The listing builds one solid part. Answer for the finished solid, in the listing's coordinates (mm). Coordinates: 2 decimals unless noted, no trailing zeros. Order: outer loops, then holes, each group sorted by start corner. A loop starts at its lowest first (then second) coordinate and runs counter-clockwise, first axis right, second up. Notation, with made-up numbers: (18, -10) - (35, -10) arc R27 ccw to (35, 16) - close; hole circle Ø11 at (-35.5, -16.5). An arc over 180 degrees is marked (long way). Use a Markdown table: item, result. Add a question column.
Item 1: The part is cut by section A-A, the plane z = -15.5. Give the vertices of the cut face in (x, y) (3 decimals), then the cut area to 3 significant figures.
Item 2: Find the intervals of material crossed by line 1 along Y through (x, z) = (-18, -4); line 2 along X through (y, z) = (-2.5, 0.5) (3 decimals); line 3 along X through (y, z) = (-10.5, 14.5) (3 decimals), in increasing order.
Item 3: The part is cut by section B-B, the plane x = -15. Give the vertices of the cut face in (y, z) (3 decimals), then the cut area to 3 significant figures.
Item 4: Flat-ended cylindrical pins translate along their axes: P1, Ø1.5, axis at x = -9.5, z = -17.5, coming from the -Y side; P2, Ø4, axis at x = 13, z = 17.5, coming from the +Y side; P3, Ø1.5, axis at x = -16, z = -2, coming from the -Y side; P4, Ø12, axis at x = -10, y = -25, coming from the +Z side (3 decimals). Find the tip coordinate at first contact, or state that the pin passes through.
from build123d import *

# Parameters (mm, degrees)
F0_W     = 44.45
F0_H     = 44.45
F1_DEPTH = 44.45
F4_DEPTH = 44.451
F5_DEPTH = 44.451


with BuildPart() as f1:
    # F0 (on Front) → F1 (new body)
    with BuildSketch(Plane.XZ):
        Rectangle(F0_W, F0_H)
    extrude(amount=F1_DEPTH)

    # F2 (on face) → F4 (cut, through all)
    with BuildSketch(Plane(origin=(-22.225, 0, 0), x_dir=(0, -1, 0), z_dir=(-1, 0, 0))):
        Polygon((44.45, 22.225), (0, 22.225), (44.45, 0), align=None)
        Polygon((44.45, -22.225), (44.45, 0), (0, -22.225), align=None)
    extrude(amount=-F4_DEPTH, mode=Mode.SUBTRACT)

    # F3 (on face) → F5 (cut, through all)
    with BuildSketch(Plane(origin=(0, 0, -22.225), x_dir=(1, 0, 0), z_dir=(0, 0, -1))):
        Polygon((22.225, 44.45), (0, 44.45), (22.225, 0), align=None)
        Polygon((-22.225, 44.45), (-22.225, 0), (0, 44.45), align=None)
    extrude(amount=-F5_DEPTH, mode=Mode.SUBTRACT)


solid = f1.part
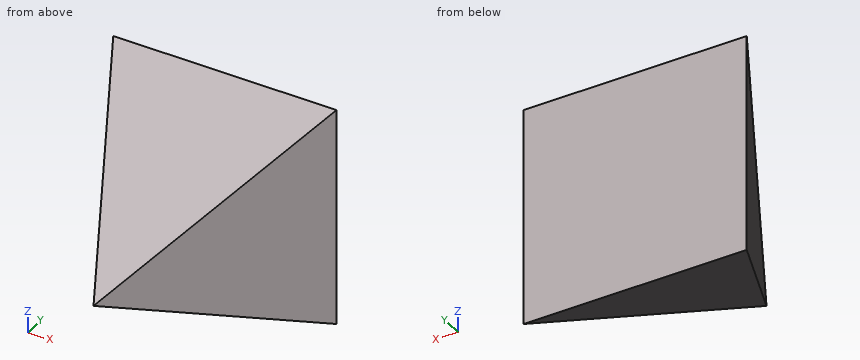
Solution:
| question | item | result |
|---|---|---|
| 1 | outline | (-22.225, 0) - (-15.5, -13.45) - (15.5, -13.45) - (22.225, 0) - close |
| 1 | area | 507 mm2 |
| 2 | line 1 | y = -8.45 to 0 |
| 2 | line 2 | x = -20.975 to 20.975 |
| 2 | line 3 | x = -16.975 to 16.975 |
| 3 | outline | (-14.45, -15) - (0, -22.225) - (0, 22.225) - (-14.45, 15) - close |
| 3 | area | 538 mm2 |
| 4 | P1 | stops at y = -10.95 |
| 4 | P2 | stops at y = 0 |
| 4 | P3 | stops at y = -13.95 |
| 4 | P4 | stops at z = 12.725 |
